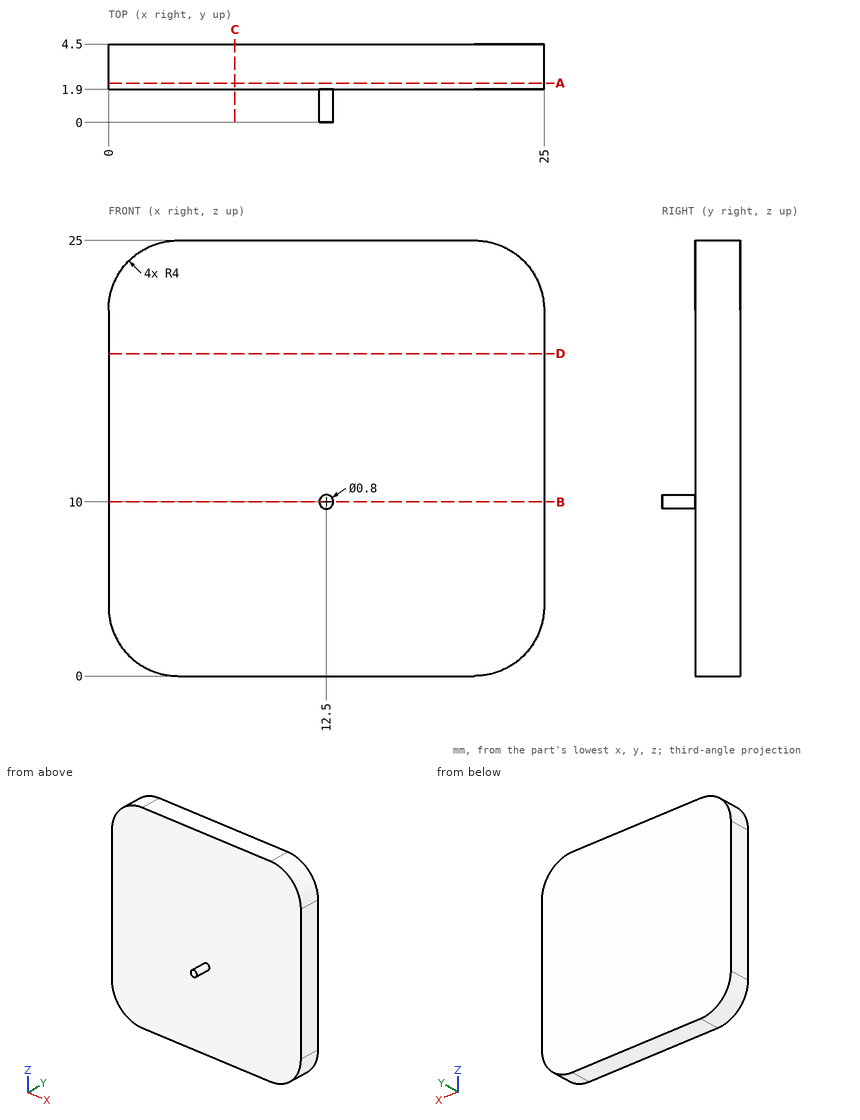
Can you work these out from the drawing? Everything is in mm from the part's minimum corner. Give positions to 0.01 mm unless a question says otherwise; leave off trailing zeros. Order: outer loops, then holes, each group sorted by start corner. A loop starts at its lowest first (then second) coordinate and runs counter-clockwise, first axis right, second up.
Item 1: If we section it at C-C, the plane x = 7.25: Write out the boundary of the cut face in (y, z).
Item 2: If we section it at A-A, the plane y = 2.25: Write out the boundary of the cut face in (x, z).
Item 3: I'm going to push a flat-ended pin straight in: pin 1 (2 mm diameter, centred on x = 21, z = 21.5, fed in from -Y). Where does the tip first touch, or does it pass through?
Item 4: If we section it at D-D, the plane z = 18.5: Write out the boundary of the cut face in (x, y), plus the area to 3 significant figures.
Item 5: If we section it at B-B, the plane z = 10: Write out the boundary of the cut face in (x, y).
Item 6: I need wall thicknesses on line 1 (Y direction, x = 17.25, z = 9); line 2 (X direction, y = 0.55, z = 10); line 3 (Z direction, x = 2, y = 3.1). Which ranges of each line are inside material? Lowest first, please.
Values:
1. outline: (1.9, 0) - (4.5, 0) - (4.5, 25) - (1.9, 25) - close
2. outline: (0, 4) arc R4 ccw to (4, 0) - (21, 0) arc R4 ccw to (25, 4) - (25, 21) arc R4 ccw to (21, 25) - (4, 25) arc R4 ccw to (0, 21) - close
3. pin 1: stops at y = 1.9
4. outline: (0, 1.9) - (25, 1.9) - (25, 4.5) - (0, 4.5) - close
4. area: 65.0 mm2
5. outline: (0, 1.9) - (12.1, 1.9) - (12.1, 0) - (12.9, 0) - (12.9, 1.9) - (25, 1.9) - (25, 4.5) - (0, 4.5) - close
6. line 1: y = 1.9 to 4.5
6. line 2: x = 12.1 to 12.9
6. line 3: z = 0.54 to 24.46
